For this review, use the dimensioned drawing (mm, ordinates from the lowest corner) and the shaded views. A direction names the side the tool comes from. Round coordinates to 2 decimals unless told otherwise and drop trailing zeros. Write each loop counter-clockwise with the first axis right and the second up, starting at its lowest first coordinate (ties: lowest second). Pieces come first, ordered by that corner, then holes. Notation, with made-up numbers: M 46.25,63.25 L 76.25,63.25 A30 cw 76.25,92.25 Z; hole C 48.5,-8.75 d11. An arc over 180 degrees is marked long. One line per question, with ' | ' between items. Start each with the question number.
Item 1: Draft analysis for pull direction X (two halves, no side actions). For the marked faces 4, 5, 6 and 7, state which applies: released by +X, released by -X, zero draft, split by the parting line, or undercut.
Item 2: Insertion check: pin 1 Ø2.5 at (y, z) = (3.5, 3) entering from +X; pin 2 Ø1.5 at (x, y) = (51.5, 16) entering from +Z; pin 3 Ø5.5 at (y, z) = (4, 2) entering from -X. Each pin has a flat end and moves straight along its axis. Give the tip position at first contact, or say it passes through.
Item 3: Add section B-B, the plane z = 27. Give the number of separate pieces and of enclosed holes in the cut face.
Item 4: Add section C-C, the plane x = 9. State the section outline as (y, z) points, and give its area (3 significant figures).
Item 5: Machinability: for the marked faces 1, 2 and 3, which of the approach directions +Z, -Z, +X, -X, +Y, -Y give a long, thin tool a straight path to every point of the face, cutting with its end or side? Answer none if there is none.
Item 6: For L1, parallel to X at y = 1, z = 3 (1 decimal); L2, parallel to Z at x = 16, y = 19.75; L3, parallel to Y at x = 19, z = 4.5, list the stretches that pass through material, from the lowest coordinate up.
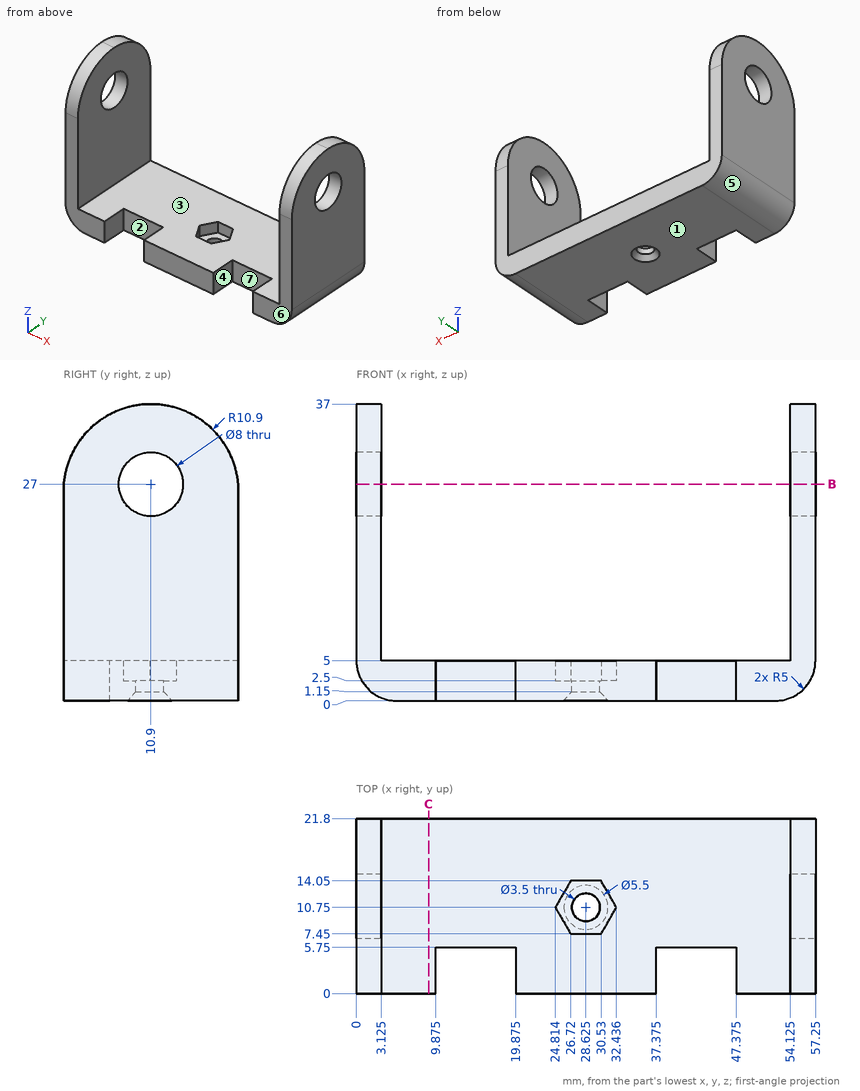
Computed values:
1) face 4: undercut | face 5: released by -X | face 6: zero draft | face 7: undercut
2) pin 1: stops at x = 57.19 | pin 2: stops at z = 5 | pin 3: stops at x = 0.01
3) separate pieces: 4 | enclosed holes: 0
4) outline: M 0,0 L 21.8,0 L 21.8,5 L 0,5 Z | area: 109 mm^2
5) face 1: -Z, +X, -X, +Y, -Y | face 2: +Z, -Z, -Y | face 3: +Z, +Y, -Y
6) L1: x = 0.4 to 9.9, 19.9 to 37.4, 47.4 to 56.8 | L2: z = 0 to 5 | L3: y = 5.75 to 21.8
